CAD build for the part. Positions are in the model's coordinates, mm. A direction names the side the tool comes from. Round coordinates to 2 decimals unless told otherwise and drop trailing zeros. Order: outer loops, then holes, each group sorted by start corner. A loop starts at its lowest first (then second) coordinate and runs counter-clockwise, first axis right, second up. Notation, with made-up numbers: (48.5, -18) - (75.5, -18) arc R30 cw to (75.5, 16) - close; hole circle Ø7 at (87, -3.75). An arc over 180 degrees is marked (long way). Use one line per item in the form item = value. Start each with the question number.
from build123d import *

# Parameters (mm, degrees)
SALIENTE_EXTRUIR1_DEPTH = 29.5
CORTAR_EXTRUIR11_DEPTH  = 18.7
CROQUIS12_W             = 20
CROQUIS12_H             = 28.5
SALIENTE_EXTRUIR2_DEPTH = 15.5
CROQUIS6_R              = 8.5
CORTAR_EXTRUIR1_DEPTH   = 10
CROQUIS7_R              = 4.1
CORTAR_EXTRUIR2_DEPTH   = 13.5
CROQUIS8_R              = 4.4
CORTAR_EXTRUIR3_DEPTH   = 6
CROQUIS2_R              = 6.1
CORTAR_EXTRUIR4_DEPTH   = 20
CORTAR_EXTRUIR5_START   = -20
CROQUIS3_R              = 6.1
CORTAR_EXTRUIR5_DEPTH   = 20
CROQUIS4_R              = 6.1
CORTAR_EXTRUIR6_DEPTH   = 20
CORTAR_EXTRUIR7_START   = -20
CROQUIS5_R              = 6.1
CORTAR_EXTRUIR7_DEPTH   = 20
CORTAR_EXTRUIR8_REACH   = 72.631
CROQUIS9_R              = 3.5
CORTAR_EXTRUIR9_REACH   = 74.107
CROQUIS10_R             = 3.5
CROQUIS13_W             = 20
CROQUIS13_H             = 24.5
CORTAR_EXTRUIR10_DEPTH  = 12.5
CORTAR_EXTRUIR12_START  = -10
CROQUIS18_R             = 1.5
CORTAR_EXTRUIR12_DEPTH  = 10
CROQUIS19_R             = 1
CORTAR_EXTRUIR13_DEPTH  = 10
CROQUIS20_R             = 2.1
CORTAR_EXTRUIR14_DEPTH  = 10


with BuildPart() as part:
    # Croquis1 → Saliente-Extruir1 (new body)
    with BuildSketch(Plane.XY):
        with BuildLine():
            Line((5.532260486, 11.858052865), (4.932758535, 18.779017183))
            Line((4.932758535, 18.779017183), (4.932758535, 36))
            ThreePointArc((4.932758535, 36), (10.243586381, 47.979347327), (21.538526154, 54.62268913))
            Line((21.538526154, 54.62268913), (23.932758535, 55))
            Line((23.932758535, 55), (56, 55))
            ThreePointArc((56, 55), (57.424264069, 54.424264069), (58, 53))
            Line((58, 53), (58, 21.932758535))
            ThreePointArc((58, 21.932758535), (50.913097547, 9.695983483), (38, 3.932758535))
            Line((38, 3.932758535), (16.641947135, 3.932758535))
            Line((16.641947135, 3.932758535), (14.26534365, 4.78116089))
            Line((14.26534365, 4.78116089), (11.904731608, 5.153727551))
            Line((11.904731608, 5.153727551), (9.720982817, 6.124570664))
            Line((9.720982817, 6.124570664), (10.875746205, 8.011278565))
            ThreePointArc((10.875746205, 8.011278565), (20.155175368, 18.125408047), (7.690637501, 12.377476547))
            Line((7.690637501, 12.377476547), (5.532260486, 11.858052865))
        make_face()
    extrude(amount=-SALIENTE_EXTRUIR1_DEPTH)

    # Croquis15 → Cortar-Extruir11 (cut)
    with BuildSketch(Plane.XY):
        with BuildLine():
            Line((58, 42.430465887), (58, 53))
            ThreePointArc((58, 53), (57.424264069, 54.424264069), (56, 55))
            Line((56, 55), (45, 55))
            Line((45, 55), (45, 54.927917446))
            ThreePointArc((45, 54.927917446), (51.043733212, 52.876346468), (54.589631863, 47.569534113))
            Line((54.589631863, 47.569534113), (58, 42.430465887))
        make_face()
    extrude(amount=-CORTAR_EXTRUIR11_DEPTH, mode=Mode.SUBTRACT)

    # Croquis12 → Saliente-Extruir2 (add)
    with BuildSketch(Plane(origin=(0, 0, -29.5), x_dir=(-1, 0, 0), z_dir=(0, 0, -1))):
        with Locations((-48, 18.25)):
            Rectangle(CROQUIS12_W, CROQUIS12_H)
    extrude(amount=-SALIENTE_EXTRUIR2_DEPTH)

    # Croquis6 → Cortar-Extruir1 (cut)
    with BuildSketch(Plane(origin=(0, 0, -29.5), x_dir=(-1, 0, 0), z_dir=(0, 0, -1))):
        with Locations((-45, 45)):
            Circle(CROQUIS6_R)
    extrude(amount=-CORTAR_EXTRUIR1_DEPTH, mode=Mode.SUBTRACT)

    # Croquis7 → Cortar-Extruir2 (cut)
    with BuildSketch(Plane(origin=(0, 0, -19.5), x_dir=(-1, 0, 0), z_dir=(0, 0, -1))):
        with Locations((-45, 45)):
            Circle(CROQUIS7_R)
    extrude(amount=-CORTAR_EXTRUIR2_DEPTH, mode=Mode.SUBTRACT)

    # Croquis8 → Cortar-Extruir3 (cut)
    with BuildSketch(Plane.XY):
        with Locations((45, 45)):
            Circle(CROQUIS8_R)
    extrude(amount=-CORTAR_EXTRUIR3_DEPTH, mode=Mode.SUBTRACT)

    # Croquis2 → Cortar-Extruir4 (cut)
    with BuildSketch(Plane.XZ.offset(-3.932758535)):
        with Locations((30, -17.5)):
            Circle(CROQUIS2_R)
    extrude(amount=-CORTAR_EXTRUIR4_DEPTH, mode=Mode.SUBTRACT)

    # Croquis3 → Cortar-Extruir5 (cut)
    with BuildSketch(Plane(origin=(0, 55, 0), x_dir=(1, 0, 0), z_dir=(0, 1, 0)).offset(CORTAR_EXTRUIR5_START)):
        with Locations((30, 17.5)):
            Circle(CROQUIS3_R)
    extrude(amount=CORTAR_EXTRUIR5_DEPTH, mode=Mode.SUBTRACT)

    # Croquis4 → Cortar-Extruir6 (cut)
    with BuildSketch(Plane.ZY.offset(-4.932758535)):
        with Locations(Location((-8.5, 30, 0), (0, 0, 270))):
            Circle(CROQUIS4_R)
    extrude(amount=-CORTAR_EXTRUIR6_DEPTH, mode=Mode.SUBTRACT)

    # Croquis5 → Cortar-Extruir7 (cut)
    with BuildSketch(Plane(origin=(58, 0, 0), x_dir=(0, 0, -1), z_dir=(1, 0, 0)).offset(CORTAR_EXTRUIR7_START)):
        with Locations(Location((8.5, 30, 0), (0, 0, 270))):
            Circle(CROQUIS5_R)
    extrude(amount=CORTAR_EXTRUIR7_DEPTH, mode=Mode.SUBTRACT)

    # Croquis9 → Cortar-Extruir8 (cut, up to next)
    with BuildSketch(Plane(origin=(38, 0, 0), x_dir=(0, 0, -1), z_dir=(1, 0, 0)), mode=Mode.PRIVATE) as cortar_extruir8_sk1:
        with Locations((8.5, 30)):
            Circle(CROQUIS9_R)
    cortar_extruir8_tool1 = extrude(cortar_extruir8_sk1.sketch, amount=-CORTAR_EXTRUIR8_REACH, mode=Mode.PRIVATE) & part.part
    add(cortar_extruir8_tool1.solids().sort_by_distance((38, 30, -8.5))[0], mode=Mode.SUBTRACT)

    # Croquis10 → Cortar-Extruir9 (cut, up to next)
    with BuildSketch(Plane.XZ.offset(-23.932758535), mode=Mode.PRIVATE) as cortar_extruir9_sk1:
        with Locations((30, -17.5)):
            Circle(CROQUIS10_R)
    cortar_extruir9_tool1 = extrude(cortar_extruir9_sk1.sketch, amount=-CORTAR_EXTRUIR9_REACH, mode=Mode.PRIVATE) & part.part
    add(cortar_extruir9_tool1.solids().sort_by_distance((30, 23.932759, -17.5))[0], mode=Mode.SUBTRACT)

    # Croquis13 → Cortar-Extruir10 (cut)
    with BuildSketch(Plane(origin=(0, 0, -29.5), x_dir=(-1, 0, 0), z_dir=(0, 0, -1))):
        with Locations((-48, 20.25)):
            Rectangle(CROQUIS13_W, CROQUIS13_H)
    extrude(amount=-CORTAR_EXTRUIR10_DEPTH, mode=Mode.SUBTRACT)

    # Croquis18 → Cortar-Extruir12 (cut)
    with BuildSketch(Plane(origin=(0, 55, 0), x_dir=(1, 0, 0), z_dir=(0, 1, 0)).offset(CORTAR_EXTRUIR12_START)):
        with Locations(Location((38.000000773, 25.50000943, 0), (0, 0, 270))):
            Circle(CROQUIS18_R)
        with Locations(Location((52.000000773, 25.50000943, 0), (0, 0, 270))):
            Circle(CROQUIS18_R)
    extrude(amount=CORTAR_EXTRUIR12_DEPTH, mode=Mode.SUBTRACT)

    # Croquis19 → Cortar-Extruir13 (cut)
    with BuildSketch(Plane(origin=(58, 0, 0), x_dir=(0, 0, -1), z_dir=(1, 0, 0))):
        with Locations((23.5, 34)):
            Circle(CROQUIS19_R)
        with Locations((23.5, 6.5)):
            Circle(CROQUIS19_R)
    extrude(amount=-CORTAR_EXTRUIR13_DEPTH, mode=Mode.SUBTRACT)

    # Croquis20 → Cortar-Extruir14 (cut)
    with BuildSketch(Plane(origin=(0, 0, -29.5), x_dir=(-1, 0, 0), z_dir=(0, 0, -1))):
        with Locations((-16, 36)):
            Circle(CROQUIS20_R)
    extrude(amount=-CORTAR_EXTRUIR14_DEPTH, mode=Mode.SUBTRACT)


solid = part.part
(1) Slice it at A-A (x = 30). Give the cut face in (y, z), and give its area (3 significant figures).
(2) Flat gauge pins, fed straight in: P1, Ø10, axis at x = 10.5, z = -21, coming from the -Y side; P2, Ø4.5, axis at x = 45, z = -24.5, coming from the -Y side. Where does each tip first touch, or does it go through?
(3) Mould opens along X. For faces 5 (the flat face through (58, 28, -15)), 6 (the cylindrical face through (47.86, 27.185, -3.088)), 7 (the cylindrical face through (16.46, 33.95, -24.57)) say: pulls with the +X half, pulls with the -X half, needs draft (parallel to the pull), parting line crosses it, or undercut.
(4) Slice it at B-B (z = -8.5). Give the number of separate pieces and of enclosed holes in the cut face, and give its area (3 significant figures).
(5) Slice it at D-D (x = 16). Give the cut face in (y, z), and give its area (3 significant figures).
(6) Which spindle directions (+Z, -Z, +X, -X, +Y, -Y) get a long thin tool onto all of the face, cutting with end or side? Do faces 1 (the cylindrical face through (33.279, 44.86, -22.644)), 2 (the flat face through (56.27, 45.04, -9.22)), 3 (the flat face through (48, 20, -17)), 4 (the flat face through (48, 4, -22)). Say none if no direction does.
(7) Wall check: line 1 (Z direction, x = 30, y = 8); line 2 (Z direction, x = 47.75, y = 30); line 3 (Y direction, x = 42.5, z = -6.5). Give the ranges that are in metal, low to high. Write a range as [from, to].
(8) Slice it at C-C (y = 29). Give the cut face in (x, z), and give its area (3 significant figures).
Results list:
q1.outline = (3.93, -29.5) - (55, -29.5) - (55, -23.6) - (35, -23.6) - (35, -21) - (23.93, -21) - (23.93, -23.6) - (3.93, -23.6) - close; (3.93, -11.4) - (23.93, -11.4) - (23.93, -14) - (35, -14) - (35, -11.4) - (55, -11.4) - (55, 0) - (3.93, 0) - close; hole circle Ø7 at (30, -8.5)
q1.area = 903 mm²
q2.P1 = 4.34
q2.P2 = 4
q3.face_5 = pulls with the +X half
q3.face_6 = needs draft
q3.face_7 = undercut
q4.separate_pieces = 2
q4.enclosed_holes = 1
q4.area = 1,630 mm²
q5.outline = (4.16, -29.5) - (7.16, -29.5) - (7.16, 0) - (4.16, 0) - close; (20.84, -29.5) - (33.9, -29.5) - (33.9, -19.5) - (38.1, -19.5) - (38.1, -29.5) - (52.54, -29.5) - (52.54, 0) - (20.84, 0) - close; hole circle Ø12.2 at (30, -8.5)
q5.area = 865 mm²
q6.face_1 = +Y
q6.face_2 = +Z, +X, +Y
q6.face_3 = -Z, +X
q6.face_4 = +Z, -Z, +X, -Y
q7.line_1 = [-29.5, -23.6], [-11.4, 0]
q7.line_2 = [-17, -14.6], [-2.4, 0]
q7.line_3 = [4.88, 24.24], [35.76, 41.75], [48.25, 55]
q8.outline = (4.93, -29.5) - (38, -29.5) - (38, -17) - (58, -17) - (58, -14.52) - (38, -14.52) - (38, -11.85) - (24.93, -11.85) - (24.93, -14.52) - (4.93, -14.52) - close; (4.93, -2.48) - (24.93, -2.48) - (24.93, -5.15) - (38, -5.15) - (38, -2.48) - (58, -2.48) - (58, 0) - (4.93, 0) - close; hole circle Ø7 at (30, -17.5)
q8.area = 708 mm²
